from build123d import *

# Parameters (mm, degrees)
BOSS_EXTRUDE1_DEPTH = 479.25
BOSS_EXTRUDE2_START = -50
SKETCH3_W           = 1980
SKETCH3_H           = 50
BOSS_EXTRUDE2_DEPTH = 58.5
FILLET1_R           = 55
BOSS_EXTRUDE4_START = -50
SKETCH4_W           = 1980
SKETCH4_H           = 50
BOSS_EXTRUDE4_DEPTH = 58.5
CUT_EXTRUDE1_START  = 529.25
SKETCH7_R           = 5.1
CUT_EXTRUDE1_DEPTH  = 50
BOSS_EXTRUDE5_START = 8.5
SKETCH8_W           = 1980
SKETCH8_H           = 24.25
SKETCH8_H_2         = 34.25
BOSS_EXTRUDE5_DEPTH = 32.7


with BuildPart() as part:
    # Sketch2 → Boss-Extrude1 (new, symmetric)
    with BuildSketch(Plane.XY):
        Polygon((-954.25, 0), (954.25, 0), (954.25, 8.5), (990, 8.5), (990, -50), (-990, -50), (-990, 8.5), (-954.25, 8.5), align=None)
    extrude(amount=BOSS_EXTRUDE1_DEPTH, both=True)

    # Sketch3 → Boss-Extrude2 (add)
    with BuildSketch(Plane(origin=(0, 0, 0), x_dir=(1, 0, 0), z_dir=(0, 1, 0)).offset(BOSS_EXTRUDE2_START)):
        with Locations((0, 504.25)):
            Rectangle(SKETCH3_W, SKETCH3_H)
    extrude(amount=BOSS_EXTRUDE2_DEPTH)

    # Fillet1
    fillet1_edges = [part.edges().sort_by_distance(p)[0] for p in [
        (954.25, 4.25, -479.25),
        (-954.25, 4.25, -479.25),
    ]]
    fillet(fillet1_edges, radius=FILLET1_R)

    # Sketch4 → Boss-Extrude4 (add)
    with BuildSketch(Plane(origin=(0, 0, 0), x_dir=(1, 0, 0), z_dir=(0, 1, 0)).offset(BOSS_EXTRUDE4_START)):
        with Locations((0, -504.25)):
            Rectangle(SKETCH4_W, SKETCH4_H)
    extrude(amount=BOSS_EXTRUDE4_DEPTH)

    # Sketch7 → Cut-Extrude1 (cut)
    with BuildSketch(Plane.XY.offset(CUT_EXTRUDE1_START)):
        with Locations((-950, 4.25)):
            Circle(SKETCH7_R)
        with Locations((950, 4.25)):
            Circle(SKETCH7_R)
    extrude(amount=-CUT_EXTRUDE1_DEPTH, mode=Mode.SUBTRACT)

    # Sketch8 → Boss-Extrude5 (add)
    with BuildSketch(Plane(origin=(0, 0, 0), x_dir=(1, 0, 0), z_dir=(0, 1, 0)).offset(BOSS_EXTRUDE5_START)):
        with Locations((0, 517.125)):
            Rectangle(SKETCH8_W, SKETCH8_H)
        with Locations((0, -512.125)):
            Rectangle(SKETCH8_W, SKETCH8_H_2)
    extrude(amount=BOSS_EXTRUDE5_DEPTH)


solid = part.part
Here's how the part is built. I have some questions about the finished solid (model axes, mm). A direction names the side the tool comes from. Give positions to 0.01 mm unless a question says otherwise; leave off trailing zeros. Write each loop counter-clockwise with the first axis right and the second up, starting at its lowest first coordinate (ties: lowest second). Pieces come first, ordered by that corner, then holes. Notation, with made-up numbers: (31, 38.25) -> (62, 38.25) arc R22 cw to (62, 69.25) -> close; hole circle Ø4 at (21, 51). An arc over 180 degrees is marked (long way). Use one line per item in the form item = value. Start each with the question number.
1. Will these pins go through, and if not, where does the flat tip stop? pin 1 Ø0.7 at (x, y) = (-954.5, 5) entering from +Z; pin 2 Ø2 at (y, z) = (11, -51) entering from -X; pin 3 Ø4.5 at (x, z) = (343, 491) entering from +Y; pin 4 Ø12 at (x, z) = (300, 353.5) entering from +Y.
2. Imagine slicing it at B-B on x = 380.5. List the corners of the cut face in (y, z) for me.
3. On a 3-axis mill with a long thin cutter (end or side, diameter ignored), from which of +Z, -Z, +X, -X, +Y, -Y can I reach the whole of each face in a straight line? I mean faces 1 (the face through (-445, 8.5, -489)), 2 (the face through (-14, -50, -7)), 3 (the face through (-937.711, 4.19, -463.566)). Say none if no direction works.
4. If I drill on L1, parallel to X at y = 4.25, z = 517; L2, parallel to Z at x = -461.5, y = 27.5; L3, parallel to Z at x = 148.5, y = 3.5, over which ranges is the centre line in solid material (lowest first)?
5. Thinking about a two-plate mould opening in Z: for faces 4 (the face through (-14, -5, -529.25)), 5 (the face through (-990, -25, 7)), 6 (the face through (938.566, 4.31, -462.711)), 7 (the face through (-13, 0, 7)), which applies, +Z half, -Z half, draft (parallel to the pull), parting line (faces both ways), or undercut?
6. Imagine slicing it at C-C on z = -336. List the corners of the cut face in (x, y) for me, plus the area to 3 significant figures.
7. Imagine slicing it at A-A on y = 26. List the corners of the cut face in (x, z) for me, plus the area to 3 significant figures.
Entries:
q1.pin_1 = 479.25
q1.pin_2 = through
q1.pin_3 = 8.5
q1.pin_4 = 0
q2.outline = (-50, -529.25) -> (41.2, -529.25) -> (41.2, -505) -> (8.5, -505) -> (8.5, -479.25) -> (0, -479.25) -> (0, 479.25) -> (8.5, 479.25) -> (8.5, 495) -> (41.2, 495) -> (41.2, 529.25) -> (-50, 529.25) -> close
q3.face_1 = +X, -X, +Y
q3.face_2 = +Z, -Z, +X, -X, -Y
q3.face_3 = +Y
q4.L1 = -990 to -955.1, -944.9 to 944.9, 955.1 to 990
q4.L2 = -529.25 to -505, 495 to 529.25
q4.L3 = -529.25 to -479.25, 479.25 to 529.25
q5.face_4 = -Z half
q5.face_5 = draft
q5.face_6 = undercut
q5.face_7 = undercut
q6.outline = (-990, -50) -> (990, -50) -> (990, 8.5) -> (954.25, 8.5) -> (954.25, 0) -> (-954.25, 0) -> (-954.25, 8.5) -> (-990, 8.5) -> close
q6.area = 99,600 mm²
q7.outline = (-990, -529.25) -> (990, -529.25) -> (990, -505) -> (-990, -505) -> close; (-990, 495) -> (990, 495) -> (990, 529.25) -> (-990, 529.25) -> close
q7.area = 116,000 mm²
